Work out the finished part from the listing and answer in its coordinate system (mm). Round coordinates to 2 decimals unless told otherwise and drop trailing zeros. Order: outer loops, then holes, each group sorted by start corner. A loop starts at its lowest first (then second) coordinate and runs counter-clockwise, first axis right, second up. Notation, with made-up numbers: (18, 13.25) -> (74, 13.25) arc R14 cw to (74, 22.25) -> close; hole circle Ø10 at (31, 73). An arc over 180 degrees is marked (long way). Use a Markdown table: item, result. Add a question column.
Item 1: A cutting plane is placed at B-B, the plane x = 56. Determine the outline of the cut face in (y, z), plus the area to 3 significant figures.
Item 2: A cutting plane is placed at A-A, the plane y = 10. Determine the outline of the cut face in (x, z), plus the area to 3 significant figures.
Item 3: Find the intervals of material crossed by L1, parallel to Y at x = -56, z = 1.15; L2, parallel to X at y = -8.25, z = 0.85; L3, parallel to X at y = -7.25, z = 0.1, in increasing order. Write a range as [from, to].
from build123d import *

# Parameters (mm, degrees)
SKETCH_1_W          = 120
SKETCH_1_H          = 30
EXTRUDE_1_DEPTH     = 3
SKETCH_3_R          = 1.5
SKETCH_3_R_2        = 1.55
CUT_EXTRUDE_2_DEPTH = 10
SKETCH_6_R          = 1.5
CUT_EXTRUDE_3_DEPTH = 10
SKETCH_8_R          = 1.55
CUT_EXTRUDE_4_DEPTH = 62.919302322


with BuildPart() as part:
    # 草图1 → 凸台-拉伸1 (new body)
    with BuildSketch(Plane.XY):
        Rectangle(SKETCH_1_W, SKETCH_1_H)
    extrude(amount=EXTRUDE_1_DEPTH)

    # 草图3 → 切除-拉伸2 (cut)
    with BuildSketch(Plane(origin=(0, 0, 0), x_dir=(-1, 0, 0), z_dir=(0, 0, -1))):
        with Locations((-56, 10)):
            Circle(SKETCH_3_R)
        with Locations((56, 10)):
            Circle(SKETCH_3_R_2)
    extrude(amount=-CUT_EXTRUDE_2_DEPTH, mode=Mode.SUBTRACT)

    # 草图6 → 切除-拉伸3 (cut)
    with BuildSketch(Plane.XY.offset(3)):
        with Locations((-56, -8)):
            Circle(SKETCH_6_R)
        with Locations((56, -8)):
            Circle(SKETCH_6_R)
    extrude(amount=-CUT_EXTRUDE_3_DEPTH, mode=Mode.SUBTRACT)

    # 草图8 → 切除-拉伸4 (cut, through all)
    with BuildSketch(Plane(origin=(0, 0, 0), x_dir=(-1, 0, 0), z_dir=(0, 0, -1))):
        with Locations((-40.146260884, 2.02)):
            Circle(SKETCH_8_R)
        with Locations((36.546260884, 2.02)):
            Circle(SKETCH_8_R)
    extrude(amount=-CUT_EXTRUDE_4_DEPTH, mode=Mode.SUBTRACT)


solid = part.part
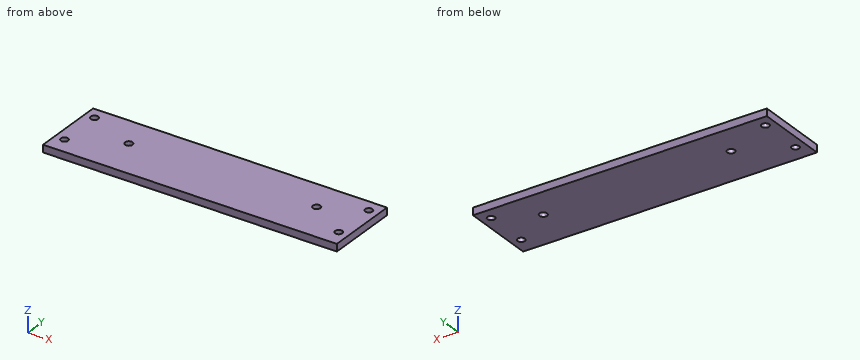
Reported:
| question | item | result |
|---|---|---|
| 1 | outline | (-15, 0) -> (-9.5, 0) -> (-9.5, 3) -> (-15, 3) -> close; (-6.5, 0) -> (8.5, 0) -> (8.5, 3) -> (-6.5, 3) -> close; (11.5, 0) -> (15, 0) -> (15, 3) -> (11.5, 3) -> close |
| 1 | area | 72.0 mm² |
| 2 | outline | (-60, 0) -> (-57.55, 0) -> (-57.55, 3) -> (-60, 3) -> close; (-54.45, 0) -> (54.5, 0) -> (54.5, 3) -> (-54.45, 3) -> close; (57.5, 0) -> (60, 0) -> (60, 3) -> (57.5, 3) -> close |
| 2 | area | 342 mm² |
| 3 | L1 | [-15, -9.5], [-6.5, 8.45], [11.55, 15] |
| 3 | L2 | [-60, -57.48], [-54.52, 54.52], [57.48, 60] |
| 3 | L3 | [-60, -57.3], [-54.7, 54.7], [57.3, 60] |
